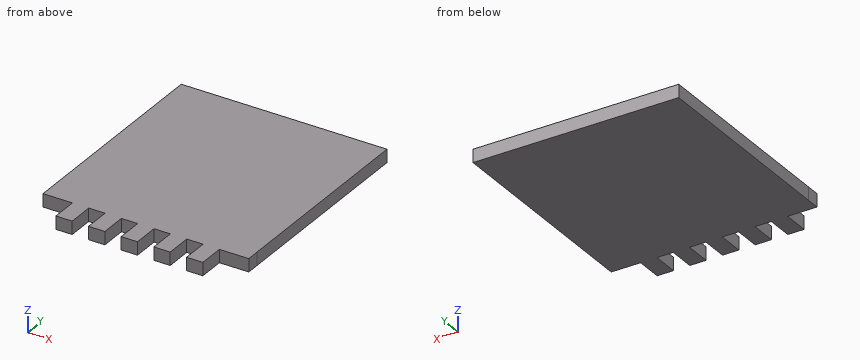
```python
from build123d import *

# Parameters (mm, degrees)
BOSS_EXTRUDE1_DEPTH = 5.08
SKETCH2_W           = 6.35
SKETCH2_H           = 10.16
SKETCH2_W_2         = 3.175
BOSS_EXTRUDE2_DEPTH = 5.08
SKETCH3_W           = 80
SKETCH3_H           = 80
BOSS_EXTRUDE3_DEPTH = 5.08


with BuildPart() as part:
    # Sketch1 → Boss-Extrude1 (new body)
    with BuildSketch(Plane.XY):
        Polygon((-32.320960724, -5.005294118), (-32.320960724, 34.994705882), (5.779039276, 34.994705882), (5.779039276, -5.005294118), (26.728959276, -5.005294118), (26.728959276, -10.085294118), (-53.271040724, -10.085294118), (-53.271040724, -5.005294118), align=None)
    extrude(amount=BOSS_EXTRUDE1_DEPTH)

    # Sketch2 → Boss-Extrude2 (add)
    with BuildSketch(Plane.XY.offset(5.08)):
        with Locations((-38.670960724, -15.165294118)):
            Rectangle(SKETCH2_W, SKETCH2_H)
        with Locations((-25.970960724, -15.165294118)):
            Rectangle(SKETCH2_W, SKETCH2_H)
        with Locations((-14.858460724, -15.165294118)):
            Rectangle(SKETCH2_W_2, SKETCH2_H)
        with Locations((-11.683460724, -15.165294118)):
            Rectangle(SKETCH2_W_2, SKETCH2_H)
        with Locations((-0.570960724, -15.165294118)):
            Rectangle(SKETCH2_W, SKETCH2_H)
        with Locations((12.129039276, -15.165294118)):
            Rectangle(SKETCH2_W, SKETCH2_H)
    extrude(amount=-BOSS_EXTRUDE2_DEPTH)

    # Sketch3 → Boss-Extrude3 (add)
    with BuildSketch(Plane.XY.offset(5.08)):
        with Locations((-13.270960724, 34.994705882)):
            Rectangle(SKETCH3_W, SKETCH3_H)
    extrude(amount=-BOSS_EXTRUDE3_DEPTH)


solid = part.part
```
Input: part model. Units: mm. Frame: model coordinates. Coordinates: 2 decimals unless noted, no trailing zeros. Order: outer loops, then holes, each group sorted by start corner. A loop starts at its lowest first (then second) coordinate and runs counter-clockwise, first axis right, second up. Notation, with made-up numbers: (-33, 81.5) - (-1, 81.5) arc R26 cw to (-1, 102.5) - close; hole circle Ø5 at (-26, 33.25). An arc over 180 degrees is marked (long way). Put each result on its own line as item: value.
1. Contact query for flat-ended pins moving along their axis: pin 1 Ø1.5 at (y, z) = (-17.5, 2.5) entering from +X; pin 2 Ø1.5 at (x, z) = (7, 3.5) entering from -Y; pin 3 Ø1.5 at (y, z) = (-16.5, 3) entering from -X. Output: stop coordinate, or through.
Report:
pin 1: stops at x = 15.3
pin 2: stops at y = -10.09
pin 3: stops at x = -41.85
2. Line query: line 1 along X through (y, z) = (-13, 3.7); line 2 along Y through (x, z) = (-31.5, 3.6). Output: solid intervals per line, ascending.
Report:
line 1: x = -41.85 to -35.5, -29.15 to -22.8, -16.45 to -10.1, -3.75 to 2.6, 8.95 to 15.3
line 2: y = -10.09 to 74.99
3. Cut plane C-C on x = -18.5. Return the cut outline in (y, z).
Report:
outline: (-10.09, 0) - (74.99, 0) - (74.99, 5.08) - (-10.09, 5.08) - close
4. Cut plane A-A on y = -14. Return the cut outline in (x, z).
Report:
outline: (-41.85, 0) - (-35.5, 0) - (-35.5, 5.08) - (-41.85, 5.08) - close; (-29.15, 0) - (-22.8, 0) - (-22.8, 5.08) - (-29.15, 5.08) - close; (-16.45, 0) - (-10.1, 0) - (-10.1, 5.08) - (-16.45, 5.08) - close; (-3.75, 0) - (2.6, 0) - (2.6, 5.08) - (-3.75, 5.08) - close; (8.95, 0) - (15.3, 0) - (15.3, 5.08) - (8.95, 5.08) - close
